Geometry check sheet. Reference: the model listing, model coordinates, mm. A direction names the side the tool comes from. Coordinates: 2 decimals unless noted, no trailing zeros. Order: outer loops, then holes, each group sorted by start corner. A loop starts at its lowest first (then second) coordinate and runs counter-clockwise, first axis right, second up. Notation, with made-up numbers: (-15.5, -31.75) -> (38.5, -31.75) arc R37 cw to (38.5, 5.25) -> close; hole circle Ø3 at (-33.75, 23.25). An arc over 180 degrees is marked (long way). Answer as CSV lines item,"result". Start each with the question number.
from build123d import *

# Parameters (mm, degrees)
SZKIC1_W                    = 20
SZKIC1_H                    = 20
SZKIC1_W_2                  = 16
SZKIC1_H_2                  = 16
SZKIC1_W_3                  = 14
SZKIC1_H_3                  = 14
DODANIE_WYCI_GNI_CIE1_DEPTH = 2
SZKIC1_4_W                  = 16
SZKIC1_4_H                  = 16
SZKIC1_4_W_2                = 14
SZKIC1_4_H_2                = 14
DODANIE_WYCI_GNI_CIE2_DEPTH = 5
ZAOKR_GLENIE1_R             = 1


with BuildPart() as part:
    # Szkic1 → Dodanie-wyci_gni_cie1 (new body)
    # profile 1 of 3: a face of its own
    with BuildSketch(Plane.XY):
        with Locations((10, 10)):
            Rectangle(SZKIC1_W, SZKIC1_H)
        with Locations((10, 10)):
            Rectangle(SZKIC1_W_2, SZKIC1_H_2, mode=Mode.SUBTRACT)
    # profile 2 of 3: a face of its own
    with BuildSketch(Plane.XY):
        with Locations((10, 10)):
            Rectangle(SZKIC1_W_2, SZKIC1_H_2)
        with Locations((10, 10)):
            Rectangle(SZKIC1_W_3, SZKIC1_H_3, mode=Mode.SUBTRACT)
    # profile 3 of 3: a face of its own
    with BuildSketch(Plane.XY):
        with Locations((10, 10)):
            Rectangle(SZKIC1_W_3, SZKIC1_H_3)
    extrude(amount=DODANIE_WYCI_GNI_CIE1_DEPTH)

    # Szkic1_4 → Dodanie-wyci_gni_cie2 (add)
    with BuildSketch(Plane.XY):
        with Locations((10, 10)):
            Rectangle(SZKIC1_4_W, SZKIC1_4_H)
        with Locations((10, 10)):
            Rectangle(SZKIC1_4_W_2, SZKIC1_4_H_2, mode=Mode.SUBTRACT)
    extrude(amount=-DODANIE_WYCI_GNI_CIE2_DEPTH)

    # Zaokr_glenie1
    zaokr_glenie1_edges = [part.edges().sort_by_distance(p)[0] for p in [
        (0, 0, 1),
        (0, 20, 1),
        (20, 20, 1),
        (20, 0, 1),
    ]]
    fillet(zaokr_glenie1_edges, radius=ZAOKR_GLENIE1_R)


solid = part.part
Q1. Sectioned sample at A-A, the plane z = -1. Record the cut outline in (x, y), then the cut area to 3 significant figures.
Q2. Thickness scan on L1, parallel to Y at x = 14.5, z = -0.25; L2, parallel to Z at x = 3, y = 1. Record the ranges inside material, lowest first.
Q3. Sectioned sample at B-B, the plane x = 9. Record the cut outline in (y, z).
Q4. Access from +Z, -Z, +X, -X, +Y, -Y to the whole of each face (thin tool, end or side, straight path). Record for faces 4 (the flat face through (17, 10, -2)), 5 (the flat face through (10, 18, -2)), 6 (the flat face through (2, 10, -2)).
Q5. Go/stop test with flat-tipped pins: pin 1 Ø2.5 at (y, z) = (9, -3.5) entering from +X; pin 2 Ø1.5 at (x, z) = (6, -1.5) entering from -Y; pin 3 Ø2.5 at (y, z) = (10, -3.5) entering from -X. Record where each tip stops, or that it passes through.
Q6. Sectioned sample at D-D, the plane x = 2.5. Record the cut outline in (y, z), then the cut area to 3 significant figures.
Q7. Release check for a two-part mould opening along Y. For faces 1 (the flat face through (18, 10, -2)), 2 (the flat face through (10, 0, 1)), 3 (the flat face through (10, 17, -2)) record: released by +Y, released by -Y, zero draft, split by the parting line, or undercut.
Geometry results:
1,outline,"(2, 2) -> (18, 2) -> (18, 18) -> (2, 18) -> close; hole (3, 3) -> (17, 3) -> (17, 17) -> (3, 17) -> close"
1,area,"60.0 mm^2"
2,L1,"y = 2 to 3, 17 to 18"
2,L2,"z = 0 to 2"
3,outline,"(0, 0) -> (2, 0) -> (2, -5) -> (3, -5) -> (3, 0) -> (17, 0) -> (17, -5) -> (18, -5) -> (18, 0) -> (20, 0) -> (20, 2) -> (0, 2) -> close"
4,face 4,"-Z"
4,face 5,"-Z, +X, -X, +Y"
4,face 6,"-Z, -X, +Y, -Y"
5,pin 1,"stops at x = 18"
5,pin 2,"stops at y = 2"
5,pin 3,"stops at x = 2"
6,outline,"(0, 0) -> (2, 0) -> (2, -5) -> (18, -5) -> (18, 0) -> (20, 0) -> (20, 2) -> (0, 2) -> close"
6,area,"120 mm^2"
7,face 1,"zero draft"
7,face 2,"released by -Y"
7,face 3,"undercut"
